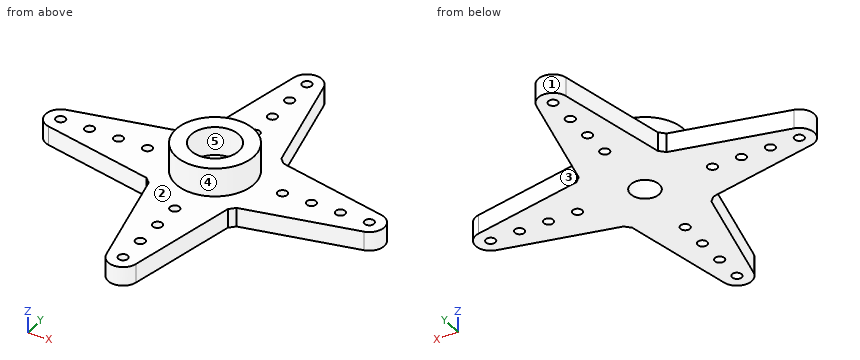
from build123d import *

# Parameters (mm, degrees)
ESQUISSE1_R                  = 1.5
ESQUISSE1_R_2                = 0.5
BOSS_EXTRU_1_DEPTH           = 2
ESQUISSE2_R                  = 4.1
ESQUISSE2_R_2                = 2.5
BOSS_EXTRU_2_DEPTH           = 3
R_P_TITION_CIRCULAIRE1_COUNT = 2
R_P_TITION_CIRCULAIRE1_ANGLE = 90


with BuildPart() as part:
    # Esquisse1 → Boss.-Extru.1 (new body)
    with BuildSketch(Plane.XY):
        with BuildLine():
            Line((-16.337044695, 1.536467752), (-4.650806382, 4.1))
            ThreePointArc((-4.650806382, 4.1), (0, 6.2), (4.650806382, 4.1))
            Line((4.650806382, 4.1), (16.337044695, 1.536467752))
            ThreePointArc((16.337044695, 1.536467752), (17.573001042, 0), (16.337044695, -1.536467752))
            Line((16.337044695, -1.536467752), (4.650806382, -4.1))
            ThreePointArc((4.650806382, -4.1), (0, -6.2), (-4.650806382, -4.1))
            Line((-4.650806382, -4.1), (-16.337044695, -1.536467752))
            ThreePointArc((-16.337044695, -1.536467752), (-17.573001042, 0), (-16.337044695, 1.536467752))
        make_face()
        Circle(ESQUISSE1_R, mode=Mode.SUBTRACT)
        with Locations((7, 0)):
            Circle(ESQUISSE1_R_2, mode=Mode.SUBTRACT)
        with Locations((16, 0)):
            Circle(ESQUISSE1_R_2, mode=Mode.SUBTRACT)
        with Locations((13, 0)):
            Circle(ESQUISSE1_R_2, mode=Mode.SUBTRACT)
        with Locations((10, 0)):
            Circle(ESQUISSE1_R_2, mode=Mode.SUBTRACT)
        with Locations((-16, 0)):
            Circle(ESQUISSE1_R_2, mode=Mode.SUBTRACT)
        with Locations((-13, 0)):
            Circle(ESQUISSE1_R_2, mode=Mode.SUBTRACT)
        with Locations((-10, 0)):
            Circle(ESQUISSE1_R_2, mode=Mode.SUBTRACT)
        with Locations((-7, 0)):
            Circle(ESQUISSE1_R_2, mode=Mode.SUBTRACT)
    boss_extru_1 = extrude(amount=BOSS_EXTRU_1_DEPTH)

    # Esquisse2 → Boss.-Extru.2 (add)
    with BuildSketch(Plane.XY.offset(2)):
        Circle(ESQUISSE2_R)
        Circle(ESQUISSE2_R_2, mode=Mode.SUBTRACT)
    extrude(amount=BOSS_EXTRU_2_DEPTH)

    # R_p_tition circulaire1: Boss.-Extru.1 ×2 about axis
    r_p_tition_circulaire1_axis = Axis((0, 0, 0), (0, 0, 1))
    for i in range(1, R_P_TITION_CIRCULAIRE1_COUNT):
        add(boss_extru_1.rotate(r_p_tition_circulaire1_axis, i * R_P_TITION_CIRCULAIRE1_ANGLE / (R_P_TITION_CIRCULAIRE1_COUNT - 1)))


solid = part.part
Work out the finished part from the listing and answer in its coordinate system (mm). Face numbers are marked on the shaded views. A direction names the side the tool comes from. Give positions to 0.01 mm unless a question says otherwise; leave off trailing zeros. Loops run counter-clockwise (first coordinate to the right, second up) from the corner with the lowest first, then second, coordinate; pieces in that order, holes last. Notation, with made-up numbers: (46.5, 87) - (58.5, 87) arc R14 cw to (58.5, 102) - close; hole circle Ø9 at (25.5, -9.5). An arc over 180 degrees is marked (long way). Answer in a Markdown table with one row per item.
(1) Section A-A (z = 0.6) is taken. State how many separate pieces and enclosed holes the cut face has, and give its area (3 significant figures).
Results list:
| item | result |
|---|---|
| separate pieces | 1 |
| enclosed holes | 17 |
| area | 341 mm² |
(2) A tool of negligible diameter and unlimited length cuts with its end or side. For the marked faces 1 and 2, from which of +Z, -Z, +X, -X, +Y, -Y can it reach the whole face along a straight path? Write none if from no direction.
Results list:
| item | result |
|---|---|
| face 1 | +Z, -Z, +Y |
| face 2 | +Z |
(3) Section C-C (y = 13) is taken. Give the vertices of the cut face in (x, z), and give its area (3 significant figures).
Results list:
| item | result |
|---|---|
| outline | (-2.27, 0) - (-0.5, 0) - (-0.5, 2) - (-2.27, 2) - close; (0.5, 0) - (2.27, 0) - (2.27, 2) - (0.5, 2) - close |
| area | 7.07 mm² |
(4) Flat-ended cylindrical pins translate along their axes: pin 1 Ø4 at (x, y) = (0, 0) entering from +Z; pin 2 Ø1 at (y, z) = (2.5, 3) entering from +X; pin 3 Ø3 at (x, z) = (-4, 4) entering from +Y. Find the tip coordinate at first contact, or state that the pin passes through.
Results list:
| item | result |
|---|---|
| pin 1 | stops at z = 2 |
| pin 2 | stops at x = 3.58 |
| pin 3 | stops at y = 3.25 |
(5) For a pull along Y with two mould halves and no side action, classify the marked faces 3, 4 and 5 as pulls with the +Y half, pulls with the -Y half, needs draft (parallel to the pull), parting line crosses it, or undercut.
Results list:
| item | result |
|---|---|
| face 3 | pulls with the +Y half |
| face 4 | parting line crosses it |
| face 5 | undercut |
(6) Section B-B (x = -10) is taken. Give the vertices of the cut face in (y, z), and give its area (3 significant figures).
Results list:
| item | result |
|---|---|
| outline | (-2.93, 0) - (-0.5, 0) - (-0.5, 2) - (-2.93, 2) - close; (0.5, 0) - (2.93, 0) - (2.93, 2) - (0.5, 2) - close |
| area | 9.71 mm² |
(7) Consider L1, parallel to Y at x = -16, z = 1.5; L2, parallel to Z at x = 15, y = 0.5; L3, parallel to X at y = 2, z = 2.2. Determine where each line is inside the solid, lowest interval first. Write a range as [from, to].
Results list:
| item | result |
|---|---|
| L1 | y = [-1.61, -0.5], [0.5, 1.61] |
| L2 | z = [0, 2] |
| L3 | x = [-3.58, -1.5], [1.5, 3.58] |
